Source: CAD feature listing. Evaluate the final solid. Frame: model axes, mm. A direction names the side the tool comes from. Round coordinates to 2 decimals unless told otherwise and drop trailing zeros. Loops run counter-clockwise (first coordinate to the right, second up) from the corner with the lowest first, then second, coordinate; pieces in that order, holes last. Notation, with made-up numbers: (61, -6.5) - (106, -6.5) arc R14 cw to (106, 12.5) - close; hole circle Ø10 at (37.25, 58.5). An arc over 180 degrees is marked (long way). One line per question, with ' | ' between items. Start each with the question number.
1. Access query for faces 1 (the flat face through (2, 5.25, 0.13)), 2 (the flat face through (1, -6, 0)). Directions: +Z, -Z, +X, -X, +Y, -Y. A direction counts if a zero-diameter tool reaches every point of the face in a straight line with its end or side. Return the directions, or none.
2. Ray query, line 1 (Y direction, x = 1.4, z = -7); line 2 (Y direction, x = 5, z = 0); line 3 (X direction, y = 1, z = -5.5). Return the intervals inside material, ascending.
3. Pin query (flat end, axial travel): pin 1 (3 mm diameter, centred on y = 0, z = -7, fed in from +X); pin 2 (2 mm diameter, centred on y = 3.5, z = -3.5, fed in from -X); pin 3 (3 mm diameter, centred on x = 7, z = -5, fed in from +Y); pin 4 (4.5 mm diameter, centred on y = 0, z = 0, fed in from +X). Return the tip coordinate at first contact, or that it passes through.
4. Cut plane B-B (x = 7.25). Return loops of the section in (y, z).
5. Cut plane A-A (z = 0). Return loops of the section in (x, y).
6. Mould query, pull axis Y, two halves, no side actions, for faces 3 (the cylindrical face through (1.14, -0.05, 5.75)), 4 (the cylindrical face through (4.996, 3.905, -0.867)), 5 (the flat face through (1, 6, 0)). Classes: pulls with the +Y half, pulls with the -Y half, needs draft (parallel to the pull), parting line crosses it, or undercut.
7. Cut plane C-C (y = 0). State how many separate pieces and enclosed holes the cut face has, then the cut area to 3 significant figures.
```python
from build123d import *

# Parameters (mm, degrees)
TROU_TARAUD_M3X0_51_AT_2_COUNT = 2
TROU_TARAUD_M3X0_51_AT_2_PITCH = 14
CHANFREIN1_SIZE                = 0.3
ESQUISSE7_W                    = 26.326678726
ESQUISSE7_H                    = 21.946612952
ESQUISSE7_W_2                  = 20
ESQUISSE7_H_2                  = 12
ENL_V_MAT_EXTRU_2_DEPTH        = 10


with BuildPart() as part:
    # Esquisse1 → Révolution1 (revolve)
    with BuildSketch(Plane.XY, mode=Mode.PRIVATE) as r_volution1_sk:
        with BuildLine():
            Line((0, 2), (8, 2))
            Line((8, 2), (8, 3.5))
            ThreePointArc((8, 3.5), (7.853553391, 3.853553391), (7.5, 4))
            Line((7.5, 4), (2.561460361, 4))
            ThreePointArc((2.561460361, 4), (1.75, 4.25), (2, 5.061460361))
            Line((2, 5.061460361), (2, 9))
            ThreePointArc((2, 9), (1.853553391, 9.353553391), (1.5, 9.5))
            Line((1.5, 9.5), (0, 9.5))
            Line((0, 9.5), (0, 2))
        make_face()
    revolve(r_volution1_sk.sketch.rotate(Axis((0, 0, 0), (1, 0, 0)), 90), axis=Axis((0, 0, 0), (1, 0, 0)))

    # Esquisse2 → Trou taraudé M3x0.51 (revolve, cut)
    with BuildSketch(Plane(origin=(0, 0, -7), x_dir=(0, 0, 1), z_dir=(0, 1, 0))):
        Polygon((0, 0), (0, 8), (1.6, 8), (1.25, 7.65), (1.25, 0), align=None)
    trou_taraud_m3x0_51 = revolve(axis=Axis((-6.35, 0, -7), (1, 0, 0)), mode=Mode.SUBTRACT)

    # Trou taraudé M3x0.51 at 2: Trou taraudé M3x0.51 ×2
    with Locations(*[(0, 0, i * TROU_TARAUD_M3X0_51_AT_2_PITCH) for i in range(1, TROU_TARAUD_M3X0_51_AT_2_COUNT)]):
        add(trou_taraud_m3x0_51, mode=Mode.SUBTRACT)

    # Chanfrein1
    chanfrein1_edges = [part.edges().sort_by_distance(p)[0] for p in [
        (0, 0, -2),
        (0, 0, 5.75),
        (0, 0, -8.25),
        (0, 0, -9.5),
        (8, 0, -2),
    ]]
    chamfer(chanfrein1_edges, length=CHANFREIN1_SIZE)

    # Esquisse7 → Enlèv. mat.-Extru.2 (cut)
    with BuildSketch(Plane(origin=(0, 0, 0), x_dir=(0, 0, -1), z_dir=(1, 0, 0))):
        Rectangle(ESQUISSE7_W, ESQUISSE7_H)
        Rectangle(ESQUISSE7_W_2, ESQUISSE7_H_2, mode=Mode.SUBTRACT)
    extrude(amount=ENL_V_MAT_EXTRU_2_DEPTH, mode=Mode.SUBTRACT)


solid = part.part
```
Answers follow:
1) face 1: +X | face 2: +Z, -Z, +X, -X, -Y
2) line 1: y = -6 to -1.25, 1.25 to 6 | line 2: y = -4 to -2, 2 to 4 | line 3: x = 0 to 2
3) pin 1: stops at x = 2 | pin 2: stops at x = 0 | pin 3: stops at y = 1.94 | pin 4: stops at x = 7.95
4) outline: circle Ø8 at (0, 0); hole circle Ø4 at (0, 0)
5) outline: (0, -6) - (2, -6) - (2, -5.06) arc R0.6 cw to (2.56, -4) - (7.5, -4) arc R0.5 ccw to (8, -3.5) - (8, -2.3) - (7.7, -2) - (0.3, -2) - (0, -2.3) - close; (0, 2.3) - (0.3, 2) - (7.7, 2) - (8, 2.3) - (8, 3.5) arc R0.5 ccw to (7.5, 4) - (2.56, 4) arc R0.6 cw to (2, 5.06) - (2, 6) - (0, 6) - close
6) face 3: undercut | face 4: parting line crosses it | face 5: pulls with the +Y half
7) separate pieces: 4 | enclosed holes: 0 | area: 42.8 mm2
